Can you work these out from the model? Positions are in its coordinate system, mm. Face numbers are marked on the shaded views. Coordinates: 2 decimals unless noted, no trailing zeros. Order: outer loops, then holes, each group sorted by start corner. A loop starts at its lowest first (then second) coordinate and runs counter-clockwise, first axis right, second up. Notation, with made-up numbers: (88.5, -13) - (92.5, -13) arc R3 cw to (92.5, -8) - close; hole circle Ø5 at (-20.5, 22). An arc over 180 degrees is marked (long way). Use a Markdown table: item, result. Add a question column.
(1) I want a section at C-C (z = -5.5). List the corners of the cut face in (x, y) for me.
(2) If I drill on L1, parallel to X at y = -9.75, z = -25.4; L2, parallel to Y at x = -25, z = -42, over which ranges is the centre line in solid material (lowest first)? Write a range as [from, to].
(3) I want a section at D-D (x = -46). List the corners of the cut face in (y, z) for me.
(4) I want a section at B-B (y = -45). List the corners of the cut face in (x, z) for me, and give its area (3 significant figures).
(5) For pin 1 Ø1.5 at (x, y) = (-13, -25) entering from +Z; pin 2 Ø15 at (x, y) = (-25.4, -25.4) entering from -Z; pin 3 Ø1.5 at (y, z) = (-44, -43.5) entering from +X, each with a flat end and sliding along its axis, tell me the tip position at first contact or that it passes through.
(6) I want a section at A-A (x = -25.4). List the corners of the cut face in (y, z) for me, and give its area (3 significant figures).
(7) We'd pull the mould along X, two halves only. Please class the marked faces 1, 2, 3 and 4: pulls with the +X half, pulls with the -X half, needs draft (parallel to the pull), parting line crosses it, or undercut.
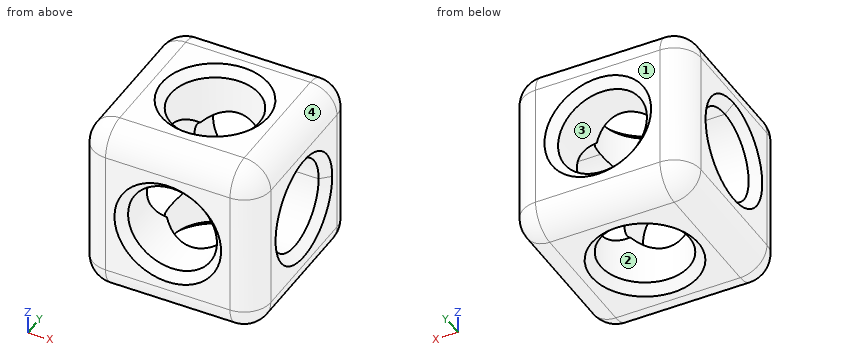
```python
from build123d import *

# Parameters (mm, degrees)
F1_DEPTH = 50.8
F2_DEPTH = 50.8
F4_DEPTH = 80.772
F6_DEPTH = 101.346
F7_R     = 7.62
F8_SIZE  = 2.54


with BuildPart() as f1:
    # F0 (on Front) → F1 (new body)
    with BuildSketch(Plane.XZ):
        Polygon((0, -50.8), (0, 0), (-50.8, 0), (-50.8, -25.4), (-50.8, -50.8), align=None)
        with BuildLine():
            ThreePointArc((-12.7, -25.4), (-25.4, -38.1), (-38.1, -25.4))
            ThreePointArc((-38.1, -25.4), (-25.4, -12.7), (-12.7, -25.4))
        make_face(mode=Mode.SUBTRACT)
    extrude(amount=F1_DEPTH)

    # F0 (on Front) → F2 (join)
    with BuildSketch(Plane.XZ):
        Polygon((0, -50.8), (0, 0), (-50.8, 0), (-50.8, -25.4), (-50.8, -50.8), align=None)
        with BuildLine():
            ThreePointArc((-12.7, -25.4), (-25.4, -38.1), (-38.1, -25.4))
            ThreePointArc((-38.1, -25.4), (-25.4, -12.7), (-12.7, -25.4))
        make_face(mode=Mode.SUBTRACT)
    extrude(amount=F2_DEPTH)

    # F3 (on face) → F4 (cut)
    with BuildSketch(Plane.XY):
        with BuildLine():
            ThreePointArc((-38.1, -25.4), (-25.4, -38.1), (-12.7, -25.4))
            ThreePointArc((-12.7, -25.4), (-25.4, -12.7), (-38.1, -25.4))
        make_face()
    extrude(amount=-F4_DEPTH, mode=Mode.SUBTRACT)

    # F5 (on face) → F6 (cut)
    with BuildSketch(Plane.YZ):
        with BuildLine():
            ThreePointArc((-25.4, -12.7), (-34.3802561211, -34.3802561211), (-12.7, -25.4))
            ThreePointArc((-12.7, -25.4), (-16.4197438789, -16.4197438789), (-25.4, -12.7))
        make_face()
    extrude(amount=-F6_DEPTH, mode=Mode.SUBTRACT)

    # F7
    f7_edges = [f1.edges().sort_by_distance(p)[0] for p in [
        (-25.4, -50.8, 0),
        (-50.8, -25.4, 0),
        (-25.4, 0, 0),
        (0, -25.4, 0),
        (0, -50.8, -25.4),
        (-25.4, -50.8, -50.8),
        (0, -25.4, -50.8),
        (0, 0, -25.4),
        (-50.8, -50.8, -25.4),
        (-50.8, -25.4, -50.8),
        (-25.4, 0, -50.8),
        (-50.8, 0, -25.4),
    ]]
    fillet(f7_edges, radius=F7_R)

    # F8
    f8_edges = [f1.edges().sort_by_distance(p)[0] for p in [
        (-38.1, -25.4, 0),
        (-38.1, -50.8, -25.4),
        (0, -38.1, -25.4),
        (-38.1, 0, -25.4),
        (-50.8, -38.1, -25.4),
        (-38.1, -25.4, -50.8),
    ]]
    chamfer(f8_edges, length=F8_SIZE)


solid = f1.part
```
Answers follow:
| question | item | result |
|---|---|---|
| 1 | outline | (-50.5, -43.18) arc R7.32 ccw to (-43.18, -50.5) - (-7.62, -50.5) arc R7.32 ccw to (-0.3, -43.18) - (-0.3, -7.62) arc R7.32 ccw to (-7.62, -0.3) - (-43.18, -0.3) arc R7.32 ccw to (-50.5, -7.62) - close; hole circle Ø25.4 at (-25.4, -25.4) |
| 2 | L1 | x = [-50.8, -38.1], [-12.7, 0] |
| 2 | L2 | y = [-50.8, -38.09], [-12.71, 0] |
| 3 | outline | (-50.26, -43.18) arc R7.08 ccw to (-43.18, -50.26) - (-7.62, -50.26) arc R7.08 ccw to (-0.54, -43.18) - (-0.54, -7.62) arc R7.08 ccw to (-7.62, -0.54) - (-43.18, -0.54) arc R7.08 ccw to (-50.26, -7.62) - close; hole circle Ø25.4 at (-25.4, -25.4) |
| 4 | outline | (-50.58, -43.18) arc R7.4 ccw to (-43.18, -50.58) - (-7.62, -50.58) arc R7.4 ccw to (-0.22, -43.18) - (-0.22, -7.62) arc R7.4 ccw to (-7.62, -0.22) - (-43.18, -0.22) arc R7.4 ccw to (-50.58, -7.62) - close; hole circle Ø25.4 at (-25.4, -25.4) |
| 4 | area | 1,980 mm² |
| 5 | pin 1 | stops at z = -2.08 |
| 5 | pin 2 | passes through |
| 5 | pin 3 | stops at x = 0 |
| 6 | outline | (-50.8, -43.18) arc R7.62 ccw to (-43.18, -50.8) - (-40.64, -50.8) - (-38.1, -48.26) - (-38.1, -38.1) - (-48.26, -38.1) - (-50.8, -40.64) - close; (-50.8, -10.16) - (-48.26, -12.7) - (-38.1, -12.7) - (-38.1, -2.54) - (-40.64, 0) - (-43.18, 0) arc R7.62 ccw to (-50.8, -7.62) - close; (-12.7, -48.26) - (-10.16, -50.8) - (-7.62, -50.8) arc R7.62 ccw to (0, -43.18) - (0, -40.64) - (-2.54, -38.1) - (-12.7, -38.1) - close; (-12.7, -12.7) - (-2.54, -12.7) - (0, -10.16) - (0, -7.62) arc R7.62 ccw to (-7.62, 0) - (-10.16, 0) - (-12.7, -2.54) - close |
| 6 | area | 570 mm² |
| 7 | face 1 | needs draft |
| 7 | face 2 | undercut |
| 7 | face 3 | undercut |
| 7 | face 4 | pulls with the +X half |
